Check sheet for the modelled part. Datum: model origin and axes. Units: mm. A direction names the side the tool comes from. Round coordinates to 2 decimals unless told otherwise and drop trailing zeros. Loops run counter-clockwise (first coordinate to the right, second up) from the corner with the lowest first, then second, coordinate; pieces in that order, holes last. Notation, with made-up numbers: (52.5, 71) - (61.5, 71) arc R15 cw to (61.5, 85) - close; hole circle Ø8 at (-38, 44.5). An arc over 180 degrees is marked (long way). Return JSON: item names as keys, results as strings.
from build123d import *

# Parameters (mm, degrees)
EXTRUDE_1_DEPTH = 2
SKETCH_2_R      = 1.5
EXTRUDE_2_DEPTH = 5


with BuildPart() as part:
    # 草图1 → 凸台-拉伸1 (new body)
    with BuildSketch(Plane(origin=(0, 0, 0), x_dir=(1, 0, 0), z_dir=(0, 1, 0))):
        Polygon((44.25, 7.5), (-44.25, 7.5), (-44.25, 3), (-53, 3), (-53, -3), (-44.25, -3), (-44.25, -7.5), (44.25, -7.5), (44.25, -3), (53, -3), (53, 3), (44.25, 3), align=None)
    extrude(amount=EXTRUDE_1_DEPTH)

    # 草图2 → 凸台-拉伸2 (add, symmetric)
    with BuildSketch(Plane.XY):
        with Locations((-53, 1)):
            Circle(SKETCH_2_R)
        with Locations((53, 1)):
            Circle(SKETCH_2_R)
    extrude(amount=EXTRUDE_2_DEPTH, both=True)


solid = part.part
Q1. Scan lines: probe 1 along X at (y, z) = (1.05, 3.5); probe 2 along X at (y, z) = (1.8, 3.75); probe 3 along X at (y, z) = (0.25, 5.25). Record each from-to range of solid material in increasing order. Write a range as [from, to].
Answer key:
{"probe 1": "x = [-54.5, -51.5], [-44.25, 44.25], [51.5, 54.5]", "probe 2": "x = [-54.27, -51.73], [-44.25, 44.25], [51.73, 54.27]", "probe 3": "x = [-44.25, 44.25]"}
Q2. Draft check along X on faces 1 (the face through (53, 1, -5)), 2 (the face through (-54.5, 1.07, -0.07)). Enter one of: released by +X, released by -X, zero draft, split by the parting line, or undercut.
Answer key:
{"face 1": "zero draft", "face 2": "undercut"}
Q3. Depth check by flat-ended pin: P1, Ø3, axis at x = -39.5, z = -5.5, coming from the +Y side; P2, Ø0.6, axis at y = 1.5, z = -5, coming from the +X side; P3, Ø0.6, axis at y = 1.5, z = 5, coming from the -X side. Enter the tip coordinate at first touch or a pass-through.
Answer key:
{"P1": "stops at y = 2", "P2": "stops at x = 54.49", "P3": "stops at x = -54.49"}
Q4. Sectioned sample at B-B (x = -53). Enter the section's corners in (y, z), plus the area to 3 significant figures.
Answer key:
{"outline": "(-0.5, -5) - (2.5, -5) - (2.5, 5) - (-0.5, 5) - close", "area": "30.0 mm²"}
Q5. Tool access check on faces 3 (the face through (44.25, 1, -5)), 4 (the face through (-44.25, 1, 5)), 5 (the face through (53, 1, 5)), 6 (the face through (-53, 1, -5)). Record the directions out of +Z, -Z, +X, -X, +Y, -Y that give a thin tool (end or side, any length) a straight path to the whole face; none if there is none.
Answer key:
{"face 3": "-Z, +Y, -Y", "face 4": "+Z, +Y, -Y", "face 5": "+Z, +X, +Y, -Y", "face 6": "-Z, -X, +Y, -Y"}
Q6. Sectioned sample at A-A (z = -4). Enter the section's corners in (x, y), plus the area to 3 significant figures.
Answer key:
{"outline": "circle Ø3 at (-53, 1); (-44.25, 0) - (44.25, 0) - (44.25, 2) - (-44.25, 2) - close; circle Ø3 at (53, 1)", "area": "191 mm²"}
